from build123d import *

# Parameters (mm, degrees)
SZKIC3_R                    = 10
DODANIE_WYCI_GNI_CIE2_DEPTH = 20


with BuildPart() as part:
    # Szkic3 → Dodanie-wyciągnięcie2 (new body)
    with BuildSketch(Plane.XY):
        with BuildLine():
            Line((12.67810929, 42.488794767), (86.036422739, 93.344089821))
            ThreePointArc((86.036422739, 93.344089821), (93.107358396, 106.849857247), (86.036422739, 120.355624672))
            Line((86.036422739, 120.355624672), (8.481056429, 156.898555423))
            Line((8.481056429, 156.898555423), (7.976636035, 180.8633929))
            Line((7.976636035, 180.8633929), (0, 180.8633929))
            Line((0, 180.8633929), (0, 199.930223275))
            Line((0, 199.930223275), (300, 200))
            Line((300, 200), (300, 180.8633929))
            Line((300, 180.8633929), (282.564213809, 180.8633929))
            Line((282.564213809, 180.8633929), (182.180079392, 75.935133422))
            Line((182.180079392, 75.935133422), (151.439346205, 55.907468715))
            Line((151.439346205, 55.907468715), (61.168077446, 12.167426414))
            ThreePointArc((61.168077446, 12.167426414), (49.626578665, 8.105505852), (37.468922524, 6.72826588))
            Line((37.468922524, 6.72826588), (25.574803596, 10.020549368))
            ThreePointArc((25.574803596, 10.020549368), (12.6494554, 18.873421693), (7.881217502, 33.796621141))
            ThreePointArc((7.881217502, 33.796621141), (9.209095866, 38.733514905), (12.67810929, 42.488794767))
        make_face()
        with Locations((29.845610796, 29.622773701)):
            Circle(SZKIC3_R, mode=Mode.SUBTRACT)
        with Locations((29.845610796, 169.541616803)):
            Circle(SZKIC3_R, mode=Mode.SUBTRACT)
    extrude(amount=DODANIE_WYCI_GNI_CIE2_DEPTH)


solid = part.part
Geometry check sheet. Reference: the model listing, model coordinates, mm. A direction names the side the tool comes from. Coordinates: 2 decimals unless noted, no trailing zeros. Order: outer loops, then holes, each group sorted by start corner. A loop starts at its lowest first (then second) coordinate and runs counter-clockwise, first axis right, second up. Notation, with made-up numbers: (-29.75, 34) - (-13.75, 34) arc R22 cw to (-13.75, 60) - close; hole circle Ø8 at (48.5, 35.5). An arc over 180 degrees is marked (long way). One line per item, written item: value.
(1) Access from +Z, -Z, +X, -X, +Y, -Y to the whole of each face (thin tool, end or side, straight path). Record for faces 4 (the face through (47.8, 138.37, 9.86)), 5 (the face through (291, 180.863, 10)), 6 (the face through (119, 126, 0)).
Data:
face 4: +Z, -Z, -X
face 5: +Z, -Z, +X, -Y
face 6: -Z, +X, -X, +Y, -Y
(2) Depth check by flat-ended pin: pin 1 Ø8 at (y, z) = (29, 12.5) entering from -X; pin 2 Ø1 at (y, z) = (149.5, 7) entering from +X; pin 3 Ø8 at (y, z) = (79.5, 9.5) entering from +X; pin 4 Ø16 at (x, y) = (29.85, 169.54) entering from -Z. Enter the tip coordinate at first touch or a pass-through.
Data:
pin 1: stops at x = 7.88
pin 2: stops at x = 253.04
pin 3: stops at x = 189.42
pin 4: passes through
(3) Thickness scan on probe 1 along X at (y, z) = (33, 10.5); probe 2 along X at (y, z) = (32, 18); probe 3 along Y at (x, z) = (69.5, 11.25). Record the ranges inside material, lowest first. Write a range as from..to.
Data:
probe 1: x = 7.88..20.43, 39.26..104.16
probe 2: x = 7.91..20.13, 39.56..102.1
probe 3: y = 16.2..81.88, 128.15..199.95
(4) Sectioned sample at C-C (y = 153.5). Enter the section's corners in (x, z), and give its area (3 significant figures).
Data:
outline: (15.69, 0) - (256.39, 0) - (256.39, 20) - (15.69, 20) - close
area: 4,810 mm^2
(5) Release check for a two-part mould opening along Y. For faces 1 (the face through (119, 126, 20)), 2 (the face through (31.61, 8.35, 9.86)), 3 (the face through (93.106, 106.628, 9.86)) record: +Y half, -Y half, draft (parallel to the pull), parting line (faces both ways), or undercut.
Data:
face 1: draft
face 2: -Y half
face 3: undercut
(6) Sectioned sample at A-A (z = 17). Enter the section's corners in (x, y).
Data:
outline: (0, 180.86) - (7.98, 180.86) - (8.48, 156.9) - (86.04, 120.36) arc R16.43 cw to (86.04, 93.34) - (12.68, 42.49) arc R10.69 ccw to (7.88, 33.8) arc R24.14 ccw to (25.57, 10.02) - (37.47, 6.73) arc R54.35 ccw to (61.17, 12.17) - (151.44, 55.91) - (182.18, 75.94) - (282.56, 180.86) - (300, 180.86) - (300, 200) - (0, 199.93) - close; hole circle Ø20 at (29.85, 29.62); hole circle Ø20 at (29.85, 169.54)
(7) Sectioned sample at B-B (x = 241.5). Enter the section's corners in (y, z).
Data:
outline: (137.94, 0) - (199.99, 0) - (199.99, 20) - (137.94, 20) - close
